Source: CAD feature listing. Evaluate the final solid. Frame: model axes, mm. Round coordinates to 2 decimals unless told otherwise and drop trailing zeros. Loops run counter-clockwise (first coordinate to the right, second up) from the corner with the lowest first, then second, coordinate; pieces in that order, holes last. Notation, with made-up numbers: (-37, 19.25) -> (-28, 19.25) arc R20 cw to (-28, 56.25) -> close; hole circle Ø8 at (47.25, 52). An arc over 180 degrees is marked (long way). Write item = value, one per line.
from build123d import *

# Parameters (mm, degrees)
BOSS_EXTRUDE1_DEPTH         = 2
BOSS_EXTRUDE1_DEPTH_BACK    = 2
SKETCH1_W                   = 130
SKETCH1_H                   = 130
TAP_DRILL_FOR_M5X0_8_TAP1_D = 5


with BuildPart() as part:
    # Sketch1 → Boss-Extrude1 (new, two sides: drawn at the far end of the back side and taken through both)
    with BuildSketch(Plane.XY.offset(-BOSS_EXTRUDE1_DEPTH_BACK)):
        Rectangle(SKETCH1_W, SKETCH1_H)
    extrude(amount=BOSS_EXTRUDE1_DEPTH + BOSS_EXTRUDE1_DEPTH_BACK)

    # Tap Drill for M5x0.8 Tap1 (through all)
    with Locations(Plane(origin=(0, 0, -2), x_dir=(-1, 0, 0), z_dir=(0, 0, -1))):
        with Locations((-56, 56), (56, 56), (56, -56), (-56, -56)):
            Hole(TAP_DRILL_FOR_M5X0_8_TAP1_D / 2)


solid = part.part
1. Mould query, pull axis Y, two halves, no side actions, for faces 1 (the face through (-1, 65, 0)), 2 (the face through (-53.69, -56.96, 0.03)), 3 (the face through (-1, 1, 2)), 4 (the face through (-53.69, 55.04, 0.03)). Classes: released by +Y, released by -Y, zero draft, split by the parting line, or undercut.
Evaluation:
face_1 = released by +Y
face_2 = undercut
face_3 = zero draft
face_4 = undercut
2. Contact query for a flat-ended pin moving along its axis: pin 1 Ø8 at (x, y) = (-56, 56) entering from -Z. Output: stop coordinate, or through.
Evaluation:
pin_1 = -2
3. Line query: probe 1 along Y at (x, z) = (56, -0.35); probe 2 along Y at (x, z) = (55, 1.5). Output: solid intervals per line, ascending. Write a range as from..to.
Evaluation:
probe_1 = -65..-58.5, -53.5..53.5, 58.5..65
probe_2 = -65..-58.29, -53.71..53.71, 58.29..65
4. Section query A-A (y = 56). Return the cut outline in (x, z), then the cut area to 3 significant figures.
Evaluation:
outline = (-65, -2) -> (-58.5, -2) -> (-58.5, 2) -> (-65, 2) -> close; (-53.5, -2) -> (53.5, -2) -> (53.5, 2) -> (-53.5, 2) -> close; (58.5, -2) -> (65, -2) -> (65, 2) -> (58.5, 2) -> close
area = 480 mm²
